```python
from build123d import *

# Parameters (mm, degrees)
SALIENTE_EXTRUIR1_DEPTH = 12.5
CROQUIS2_R              = 1.7
CORTAR_EXTRUIR1_DEPTH   = 9
CROQUIS6_R              = 3.1
CORTAR_EXTRUIR4_DEPTH   = 3
REDONDEO1_R             = 3


with BuildPart() as part:
    # Croquis1 → Saliente-Extruir1 (new body, symmetric)
    with BuildSketch(Plane.XY):
        with BuildLine():
            Line((-16.5, 7.5), (-8.440971508, 7.5))
            ThreePointArc((-8.440971508, 7.5), (0, 0), (8.440971508, 7.5))
            Line((8.440971508, 7.5), (16.5, 7.5))
            Line((16.5, 7.5), (16.5, -1.5))
            Line((16.5, -1.5), (8.306623863, -1.5))
            ThreePointArc((8.306623863, -1.5), (0, -4.5), (-8.306623863, -1.5))
            Line((-8.306623863, -1.5), (-16.5, -1.5))
            Line((-16.5, -1.5), (-16.5, 7.5))
        make_face()
    extrude(amount=SALIENTE_EXTRUIR1_DEPTH, both=True)

    # Croquis2 → Cortar-Extruir1 (cut)
    with BuildSketch(Plane(origin=(0, 7.5, 0), x_dir=(1, 0, 0), z_dir=(0, 1, 0))):
        with Locations((-12.470485754, 6.25)):
            Circle(CROQUIS2_R)
        with Locations((12.470485754, 6.25)):
            Circle(CROQUIS2_R)
        with Locations((12.470485754, -6.25)):
            Circle(CROQUIS2_R)
        with Locations((-12.470485754, -6.25)):
            Circle(CROQUIS2_R)
    extrude(amount=-CORTAR_EXTRUIR1_DEPTH, mode=Mode.SUBTRACT)

    # Croquis6 → Cortar-Extruir4 (cut)
    with BuildSketch(Plane.XZ.offset(1.5)):
        with Locations((-12.470485754, 6.25)):
            Circle(CROQUIS6_R)
        with Locations((12.470485754, 6.25)):
            Circle(CROQUIS6_R)
        with Locations((12.470485754, -6.25)):
            Circle(CROQUIS6_R)
        with Locations((-12.470485754, -6.25)):
            Circle(CROQUIS6_R)
    extrude(amount=-CORTAR_EXTRUIR4_DEPTH, mode=Mode.SUBTRACT)

    # Redondeo1
    redondeo1_edges = [part.edges().sort_by_distance(p)[0] for p in [
        (16.5, 3, -12.5),
        (-16.5, 3, 12.5),
        (16.5, 3, 12.5),
        (-16.5, 3, -12.5),
    ]]
    fillet(redondeo1_edges, radius=REDONDEO1_R)


solid = part.part
```
Here's how the part is built. I have some questions about the finished solid (model axes, mm). A direction names the side the tool comes from. Give positions to 0.01 mm unless a question says otherwise; leave off trailing zeros. Loops run counter-clockwise (first coordinate to the right, second up) from the corner with the lowest first, then second, coordinate; pieces in that order, holes last. Notation, with made-up numbers: (8, 84.5) -> (29, 84.5) arc R16 cw to (29, 102.5) -> close; hole circle Ø6 at (45, 49.25). An arc over 180 degrees is marked (long way). Use one line per item in the form item = value. Start each with the question number.
1) For P1, Ø5, axis at x = 12.5, z = -6.5, coming from the -Y side; P2, Ø4, axis at x = 13, z = 4, coming from the -Y side, each with a flat end and sliding along its axis, tell me the tip position at first contact or that it passes through.
2) Imagine slicing it at C-C (z = -0.5). Please give me the cut outline in (x, y), then the cut area to 3 significant figures.
3) Which directions (+Z, -Z, +X, -X, +Y, -Y) give clear straight access to the entire face, cutting with the end or side of a thin tool? Please do faces 5 (the face through (12, -1.5, 0)), 6 (the face through (-12, -1.5, 0)), 7 (the face through (-11, 1.5, -8)), 8 (the face through (-11.69, 4.54, 7.76)), 9 (the face through (15.6, 2.94, 11.64)).
4) Thinking about a two-plate mould opening in Z: for faces 1 (the face through (14, 1.5, -8)), 2 (the face through (0, -1, 12.5)), 3 (the face through (9.373, -0.021, -6.114)), 4 (the face through (12, 7.5, 0)), which applies, +Z half, -Z half, draft (parallel to the pull), parting line (faces both ways), or undercut?
5) Imagine slicing it at B-B (z = -6.25). Please give me the cut outline in (x, y).
6) Please list where these lines run through material, in increasing order: line 1 along Z through (x, y) = (-12, 5); line 2 along X through (y, z) = (3.9, -6.25); line 3 along X through (y, z) = (5.35, -6.25).
7) Imagine slicing it at A-A (y = 6.25). Please give me the cut outline in (x, z).
8) Imagine slicing it at D-D (y = 0.5). Please give me the cut outline in (x, z).
Check values:
q1.P1 = 1.5
q1.P2 = -1.5
q2.outline = (-16.5, -1.5) -> (-8.31, -1.5) arc R13 ccw to (8.31, -1.5) -> (16.5, -1.5) -> (16.5, 7.5) -> (8.44, 7.5) arc R8.5 cw to (-8.44, 7.5) -> (-16.5, 7.5) -> close
q2.area = 235 mm^2
q3.face_5 = +Z, -Z, +X, -Y
q3.face_6 = +Z, -Z, -X, -Y
q3.face_7 = -Y
q3.face_8 = +Y, -Y
q3.face_9 = +Z, +X, +Y, -Y
q4.face_1 = undercut
q4.face_2 = +Z half
q4.face_3 = undercut
q4.face_4 = draft
q5.outline = (-16.5, -1.5) -> (-15.57, -1.5) -> (-15.57, 1.5) -> (-14.17, 1.5) -> (-14.17, 7.5) -> (-16.5, 7.5) -> close; (-10.77, 1.5) -> (-9.37, 1.5) -> (-9.37, -1.5) -> (-8.31, -1.5) arc R13 ccw to (8.31, -1.5) -> (9.37, -1.5) -> (9.37, 1.5) -> (10.77, 1.5) -> (10.77, 7.5) -> (8.44, 7.5) arc R8.5 cw to (-8.44, 7.5) -> (-10.77, 7.5) -> close; (14.17, 1.5) -> (15.57, 1.5) -> (15.57, -1.5) -> (16.5, -1.5) -> (16.5, 7.5) -> (14.17, 7.5) -> close
q6.line_1 = -12.5 to -7.88, -4.62 to 4.62, 7.88 to 12.5
q6.line_2 = -16.5 to -14.17, -10.77 to -7.15, 7.15 to 10.77, 14.17 to 16.5
q6.line_3 = -16.5 to -14.17, -10.77 to -7.89, 7.89 to 10.77, 14.17 to 16.5
q7.outline = (-16.5, -9.5) arc R3 ccw to (-13.5, -12.5) -> (-8.2, -12.5) -> (-8.2, 12.5) -> (-13.5, 12.5) arc R3 ccw to (-16.5, 9.5) -> close; (8.2, -12.5) -> (13.5, -12.5) arc R3 ccw to (16.5, -9.5) -> (16.5, 9.5) arc R3 ccw to (13.5, 12.5) -> (8.2, 12.5) -> close; hole circle Ø3.4 at (-12.47, -6.25); hole circle Ø3.4 at (-12.47, 6.25); hole circle Ø3.4 at (12.47, -6.25); hole circle Ø3.4 at (12.47, 6.25)
q8.outline = (-16.5, -9.5) arc R3 ccw to (-13.5, -12.5) -> (-2.87, -12.5) -> (-2.87, 12.5) -> (-13.5, 12.5) arc R3 ccw to (-16.5, 9.5) -> close; (2.87, -12.5) -> (13.5, -12.5) arc R3 ccw to (16.5, -9.5) -> (16.5, 9.5) arc R3 ccw to (13.5, 12.5) -> (2.87, 12.5) -> close; hole circle Ø6.2 at (-12.47, -6.25); hole circle Ø6.2 at (-12.47, 6.25); hole circle Ø6.2 at (12.47, -6.25); hole circle Ø6.2 at (12.47, 6.25)
